Design review of the part built by this model. Coordinates are the model's own, in mm. Coordinates: 2 decimals unless noted, no trailing zeros. Order: outer loops, then holes, each group sorted by start corner. A loop starts at its lowest first (then second) coordinate and runs counter-clockwise, first axis right, second up. Notation, with made-up numbers: (-36.75, -33.75) -> (-3.75, -33.75) arc R21 ccw to (-3.75, 3.25) -> close; hole circle Ø8 at (88, -7). An arc over 180 degrees is marked (long way). Write item = value, one per line.
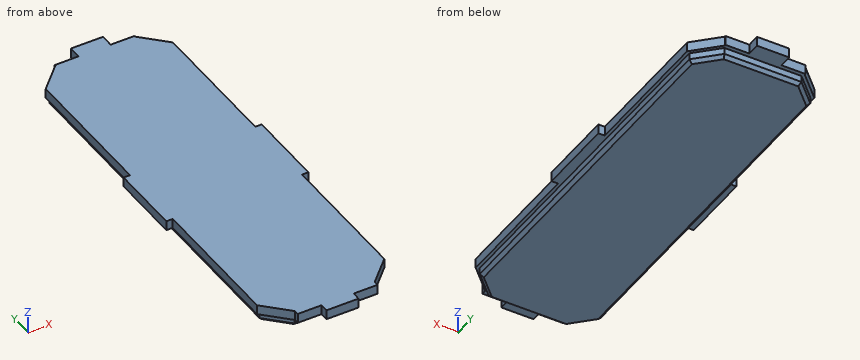
```python
from build123d import *

# Parameters (mm, degrees)
BOSS_EXTRUDE1_DEPTH = 1.5
BOSS_EXTRUDE2_DEPTH = 1.5
SKETCH3_W           = 2
SKETCH3_H           = 12.202692118
SKETCH3_H_2         = 11.147562167
BOSS_EXTRUDE3_DEPTH = 1.5
CHAMFER2_SIZE       = 0.5


with BuildPart() as part:
    # Sketch1 → Boss-Extrude1 (new body)
    with BuildSketch(Plane.XY):
        Polygon((-135.194999999, -141.317867967), (-131.782867965, -144.730000001), (-119.797132034, -144.730000001), (-116.384999999, -141.317867967), (-116.384999999, -86.586255973), (-119.797132034, -83.174123939), (-131.782867965, -83.174123939), (-135.194999999, -86.586255973), align=None)
    extrude(amount=-BOSS_EXTRUDE1_DEPTH)

    # Sketch2 → Boss-Extrude2 (add)
    with BuildSketch(Plane.XY):
        Polygon((-135.694999999, -86.379149192), (-135.694999999, -141.524974748), (-131.989974746, -145.230000001), (-119.590025252, -145.230000001), (-115.884999999, -141.524974748), (-115.884999999, -86.379149192), (-119.590025252, -82.674123939), (-131.989974746, -82.674123939), align=None)
    extrude(amount=BOSS_EXTRUDE2_DEPTH)

    # Sketch3 → Boss-Extrude3 (add)
    with BuildSketch(Plane.XY.offset(1.5)):
        Polygon((-131.989974746, -83.526014077), (-128.289999999, -83.526014077), (-128.289999999, -84.5222338), (-123.289999999, -84.5222338), (-123.289999999, -83.526014077), (-119.590025252, -83.526014077), (-119.590025252, -82.5222338), (-123.289999999, -82.5222338), (-123.289999999, -80.5222338), (-128.289999999, -80.5222338), (-128.289999999, -82.5222338), (-131.989974746, -82.5222338), align=None)
        Polygon((-131.989974746, -143.816923353), (-128.289999999, -143.816923353), (-128.289999999, -143.230000001), (-123.289999999, -143.230000001), (-123.289999999, -143.816923353), (-119.590025252, -143.816923353), (-119.590025252, -145.943076649), (-123.289999999, -145.943076649), (-123.289999999, -147.230000001), (-128.289999999, -147.230000001), (-128.289999999, -145.943076649), (-131.989974746, -145.943076649), align=None)
        with Locations((-115.884999999, -113.95206197)):
            Rectangle(SKETCH3_W, SKETCH3_H)
        with Locations((-135.694999999, -113.95206197)):
            Rectangle(SKETCH3_W, SKETCH3_H_2)
    extrude(amount=-BOSS_EXTRUDE3_DEPTH)

    # Chamfer2
    chamfer2_edges = [part.edges().sort_by_distance(p)[0] for p in [
        (-125.789999999, -144.730000001, -1.5),
        (-118.091066016, -143.023933984, -1.5),
        (-116.384999999, -113.95206197, -1.5),
        (-118.091066016, -84.880189956, -1.5),
        (-125.789999999, -83.174123939, -1.5),
        (-133.488933982, -84.880189956, -1.5),
        (-135.194999999, -113.95206197, -1.5),
        (-133.488933982, -143.023933984, -1.5),
    ]]
    chamfer(chamfer2_edges, length=CHAMFER2_SIZE)


solid = part.part
```
(1) Insertion check: pin 1 (1.1 mm diameter, centred on x = -136, z = 0.5, fed in from -Y); pin 2 (0.8 mm diameter, centred on y = -107.5, z = -0.5, fed in from +X) (3 decimals); pin 3 (0.8 mm diameter, centred on x = -121, z = 0.5, fed in from -Y). Each pin has a flat end and moves straight along its axis. Give the tip position at first contact, or say it passes through.
Report:
pin_1 = -141.77
pin_2 = -116.385
pin_3 = -145.94
(2) We need section B-B (z = -0.5). Write out the cut boundary in (x, y) (3 decimals), and give its area (3 significant figures).
Report:
outline = (-135.195, -141.318) -> (-131.783, -144.73) -> (-119.797, -144.73) -> (-116.385, -141.318) -> (-116.385, -86.586) -> (-119.797, -83.174) -> (-131.783, -83.174) -> (-135.195, -86.586) -> close
area = 1,130 mm²
(3) We need section C-C (x = -125.5). Write out the cut boundary in (y, z), and give its area (3 significant figures).
Report:
outline = (-147.23, 0) -> (-144.73, 0) -> (-144.73, -1) -> (-144.23, -1.5) -> (-83.67, -1.5) -> (-83.17, -1) -> (-83.17, 0) -> (-80.52, 0) -> (-80.52, 1.5) -> (-147.23, 1.5) -> close
area = 192 mm²
(4) For L1, parallel to X at y = -139.5, z = 0.6 (3 decimals); L2, parallel to X at y = -120, z = -0.65 (3 decimals); L3, parallel to Y at x = -128.75, z = 0.3, list the stretches that pass through material, from the lowest coordinate up.
Report:
L1 = -135.695 to -115.885
L2 = -135.195 to -116.385
L3 = -145.94 to -82.52
(5) We need section A-A (y = -111). Write out the cut boundary in (x, z) (3 decimals), and give its area (3 significant figures).
Report:
outline = (-136.695, 0) -> (-135.195, 0) -> (-135.195, -1) -> (-134.695, -1.5) -> (-116.885, -1.5) -> (-116.385, -1) -> (-116.385, 0) -> (-114.885, 0) -> (-114.885, 1.5) -> (-136.695, 1.5) -> close
area = 60.7 mm²
